Could you check a few things on this model? Use its own coordinates, in mm. A direction names the side the tool comes from. Give positions to 0.01 mm unless a question says otherwise; leave off trailing zeros. Order: outer loops, then holes, each group sorted by start corner. A loop starts at its lowest first (then second) coordinate and runs counter-clockwise, first axis right, second up. Notation, with made-up numbers: (83.5, 85) - (108.5, 85) arc R18 ccw to (108.5, 102) - close; hole circle Ø2 at (20.5, 78.5). An arc over 180 degrees is marked (long way). Put each result on its own line as item: value.
from build123d import *

# Parameters (mm, degrees)
SKETCH1_W           = 53
SKETCH1_H           = 61
BOSS_EXTRUDE1_DEPTH = 5
SKETCH2_W           = 5
SKETCH2_H           = 34
BOSS_EXTRUDE2_DEPTH = 5
SKETCH3_W           = 53
SKETCH3_H           = 5
BOSS_EXTRUDE3_DEPTH = 3
SKETCH4_W           = 53
SKETCH4_H           = 3
BOSS_EXTRUDE4_DEPTH = 8
SKETCH5_W           = 53
SKETCH5_H           = 3
BOSS_EXTRUDE5_DEPTH = 3
CUT_EXTRUDE1_REACH  = 83.847
SKETCH6_W           = 19.5
SKETCH6_H           = 6
CHAMFER1_SIZE       = 0.5
FILLET1_R           = 2.5
SKETCH7_R           = 15
CUT_EXTRUDE2_DEPTH  = 5
FILLET2_R           = 3
SKETCH8_W           = 39
SKETCH8_H           = 3
BOSS_EXTRUDE6_DEPTH = 3
SKETCH10_R          = 1.9
BOSS_EXTRUDE7_DEPTH = 4
FILLET3_START       = 4
FILLET3_DEPTH       = 2
FILLET3_2_DEPTH     = 5
FILLET3_START_2     = 10
FILLET3_3_DEPTH     = 34.381943016
SKETCH11_R          = 1.9
CUT_EXTRUDE3_DEPTH  = 5


with BuildPart() as part:
    # Sketch1 → Boss-Extrude1 (new body)
    with BuildSketch(Plane(origin=(0, 0, 0), x_dir=(1, 0, 0), z_dir=(0, 1, 0))):
        with Locations((26.5, -30.5)):
            Rectangle(SKETCH1_W, SKETCH1_H)
    extrude(amount=BOSS_EXTRUDE1_DEPTH)

    # Sketch2 → Boss-Extrude2 (add)
    with BuildSketch(Plane(origin=(0, 5, 0), x_dir=(1, 0, 0), z_dir=(0, 1, 0))):
        with Locations((2.5, -27)):
            Rectangle(SKETCH2_W, SKETCH2_H)
        with Locations((50.5, -27)):
            Rectangle(SKETCH2_W, SKETCH2_H)
    extrude(amount=BOSS_EXTRUDE2_DEPTH)

    # Sketch3 → Boss-Extrude3 (add)
    with BuildSketch(Plane(origin=(0, 0, 0), x_dir=(-1, 0, 0), z_dir=(0, 0, -1))):
        with Locations((-26.5, 2.5)):
            Rectangle(SKETCH3_W, SKETCH3_H)
    extrude(amount=BOSS_EXTRUDE3_DEPTH)

    # Sketch4 → Boss-Extrude4 (add)
    with BuildSketch(Plane(origin=(0, 5, 0), x_dir=(1, 0, 0), z_dir=(0, 1, 0))):
        with Locations((26.5, 1.5)):
            Rectangle(SKETCH4_W, SKETCH4_H)
    extrude(amount=BOSS_EXTRUDE4_DEPTH)

    # Sketch5 → Boss-Extrude5 (add)
    with BuildSketch(Plane.XY):
        with Locations((26.5, 11.5)):
            Rectangle(SKETCH5_W, SKETCH5_H)
    extrude(amount=BOSS_EXTRUDE5_DEPTH)

    # Cut-Extrude1: up to this face of the body (flat: up to its plane)
    cut_extrude1_end = Plane(part.part.faces().sort_by_distance((26.5, 5, 30.911337712))[0])
    # Sketch6 → Cut-Extrude1 (cut, up to the picked face)
    with BuildSketch(Plane(origin=(0, 13, 0), x_dir=(1, 0, 0), z_dir=(0, 1, 0)), mode=Mode.PRIVATE) as cut_extrude1_sk1:
        with Locations((36.25, 0)):
            Rectangle(SKETCH6_W, SKETCH6_H)
    cut_extrude1_tool1 = split(extrude(cut_extrude1_sk1.sketch, amount=-CUT_EXTRUDE1_REACH, mode=Mode.PRIVATE), bisect_by=cut_extrude1_end, keep=Keep.BOTH, mode=Mode.PRIVATE)
    # Sketch6 → Cut-Extrude1 (cut, up to the picked face)
    with BuildSketch(Plane(origin=(0, 13, 0), x_dir=(1, 0, 0), z_dir=(0, 1, 0)), mode=Mode.PRIVATE) as cut_extrude1_sk2:
        with Locations((16.75, 0)):
            Rectangle(SKETCH6_W, SKETCH6_H)
    cut_extrude1_tool2 = split(extrude(cut_extrude1_sk2.sketch, amount=-CUT_EXTRUDE1_REACH, mode=Mode.PRIVATE), bisect_by=cut_extrude1_end, keep=Keep.BOTH, mode=Mode.PRIVATE)
    add(cut_extrude1_tool1.solids().sort_by(Axis((36.25, 13, 0), (0, -1, 0)))[0], mode=Mode.SUBTRACT)
    add(cut_extrude1_tool2.solids().sort_by(Axis((16.75, 13, 0), (0, -1, 0)))[0], mode=Mode.SUBTRACT)

    # Chamfer1
    chamfer1_edges = [part.edges().sort_by_distance(p)[0] for p in [
        (2.5, 10, 10),
        (2.5, 10, 44),
        (50.5, 10, 44),
        (50.5, 10, 10),
    ]]
    chamfer(chamfer1_edges, length=CHAMFER1_SIZE)

    # Fillet1
    fillet1_edges = [part.edges().sort_by_distance(p)[0] for p in [
        (3.5, 13, -3),
        (49.5, 13, -3),
    ]]
    fillet(fillet1_edges, radius=FILLET1_R)

    # Sketch7 → Cut-Extrude2 (cut)
    with BuildSketch(Plane(origin=(0, 5, 0), x_dir=(1, 0, 0), z_dir=(0, 1, 0))):
        with Locations(Location((26.5, -22, 0), (0, 0, 270))):
            Circle(SKETCH7_R)
    extrude(amount=-CUT_EXTRUDE2_DEPTH, mode=Mode.SUBTRACT)

    # Fillet2
    fillet2_edges = [part.edges().sort_by_distance(p)[0] for p in [
        (53, 2.5, 61),
        (0, 2.5, 61),
    ]]
    fillet(fillet2_edges, radius=FILLET2_R)

    # Sketch8 → Boss-Extrude6 (add)
    with BuildSketch(Plane(origin=(0, 5, 0), x_dir=(1, 0, 0), z_dir=(0, 1, 0))):
        with Locations((26.5, 1.5)):
            Rectangle(SKETCH8_W, SKETCH8_H)
    extrude(amount=BOSS_EXTRUDE6_DEPTH)

    # Sketch10 → Boss-Extrude7 (add)
    # profile 1 of 2: a face of its own
    with BuildSketch(Plane.XZ):
        with BuildLine():
            Line((53, 12.5), (53, 42.5))
            ThreePointArc((53, 42.5), (68, 27.5), (53, 12.5))
        make_face()
        with Locations(Location((61, 27.5, 0), (0, 0, 90))):
            Circle(SKETCH10_R, mode=Mode.SUBTRACT)
    # profile 2 of 2: a face of its own
    with BuildSketch(Plane.XZ):
        with BuildLine():
            Line((0, 12.5), (0, 42.5))
            ThreePointArc((0, 42.5), (-15, 27.5), (0, 12.5))
        make_face()
        with Locations(Location((-8, 27.5, 0), (0, 0, 270))):
            Circle(SKETCH10_R, mode=Mode.SUBTRACT)
    extrude(amount=-BOSS_EXTRUDE7_DEPTH)

    # Fillet3: read off the stored shape, not the designer's step
    # Fillet3 outline → Fillet3 (add)
    with BuildSketch(Plane(origin=(0, 0, 0), x_dir=(1, 0, 0), z_dir=(0, 1, 0)).offset(FILLET3_START)):
        with BuildLine():
            ThreePointArc((0, -10.618056984), (-0.504909997, -11.946479312), (-1.764705882, -12.604167927))
            ThreePointArc((-1.764705882, -12.604167927), (-15, -27.5), (-1.764705882, -42.395832073))
            ThreePointArc((-1.764705882, -42.395832073), (-0.639238058, -42.916225808), (-0.03680884, -44))
            Line((-0.03680884, -44), (0, -44))
            Line((0, -44), (0, -10.618056984))
        make_face()
        with BuildLine():
            Line((53, -44), (53.03680884, -44))
            ThreePointArc((53.03680884, -44), (53.639238058, -42.916225808), (54.764705882, -42.395832073))
            ThreePointArc((54.764705882, -42.395832073), (68, -27.5), (54.764705882, -12.604167927))
            ThreePointArc((54.764705882, -12.604167927), (53.504909997, -11.946479312), (53, -10.618056984))
            Line((53, -10.618056984), (53, -44))
        make_face()
    extrude(amount=FILLET3_DEPTH)

    # Fillet3 2 outline → Fillet3 2 (add)
    with BuildSketch(Plane(origin=(0, 0, 0), x_dir=(1, 0, 0), z_dir=(0, 1, 0))):
        with BuildLine():
            Line((0, -12.5), (0, -10.618056984))
            ThreePointArc((0, -10.618056984), (-0.504909997, -11.946479312), (-1.764705882, -12.604167927))
            ThreePointArc((-1.764705882, -12.604167927), (-0.883888823, -12.526064627), (0, -12.5))
        make_face()
        with BuildLine():
            ThreePointArc((0, -42.5), (-0.883888823, -42.473935373), (-1.764705882, -42.395832073))
            ThreePointArc((-1.764705882, -42.395832073), (-0.504909997, -43.053520688), (0, -44.381943016))
            Line((0, -44.381943016), (0, -42.5))
        make_face()
        with BuildLine():
            ThreePointArc((53, -44.381943016), (53.504909997, -43.053520688), (54.764705882, -42.395832073))
            ThreePointArc((54.764705882, -42.395832073), (53.883888823, -42.473935373), (53, -42.5))
            Line((53, -42.5), (53, -44.381943016))
        make_face()
        with BuildLine():
            ThreePointArc((53, -12.5), (53.883888823, -12.526064627), (54.764705882, -12.604167927))
            ThreePointArc((54.764705882, -12.604167927), (53.504909997, -11.946479312), (53, -10.618056984))
            Line((53, -10.618056984), (53, -12.5))
        make_face()
    extrude(amount=FILLET3_2_DEPTH)

    # Fillet3 3 outline → Fillet3 3 (cut)
    with BuildSketch(Plane.XY.offset(FILLET3_START_2)):
        with BuildLine():
            Line((-16, 4), (-2, 4))
            ThreePointArc((-2, 4), (-0.585786438, 4.585786438), (0, 6))
            Line((0, 6), (-16, 6))
            Line((-16, 6), (-16, 4))
        make_face()
        with BuildLine():
            ThreePointArc((53, 6), (53.585786438, 4.585786438), (55, 4))
            Line((55, 4), (69, 4))
            Line((69, 4), (69, 6))
            Line((69, 6), (53, 6))
        make_face()
    extrude(amount=FILLET3_3_DEPTH, mode=Mode.SUBTRACT)

    # Sketch11 → Cut-Extrude3 (cut)
    with BuildSketch(Plane(origin=(0, 5, 0), x_dir=(1, 0, 0), z_dir=(0, 1, 0))):
        with Locations(Location((5, -57.5, 0), (0, 0, 270))):
            Circle(SKETCH11_R)
        with Locations(Location((48, -57.5, 0), (0, 0, 270))):
            Circle(SKETCH11_R)
    extrude(amount=-CUT_EXTRUDE3_DEPTH, mode=Mode.SUBTRACT)


solid = part.part
1) Suppose I cut it at D-D, the plane x = 44. List the corners of the cut face in (y, z) for me, and give its area (3 significant figures).
Filled in:
outline: (0, -3) - (8, -3) - (8, 0) - (5, 0) - (5, 61) - (0, 61) - close
area: 329 mm^2
2) Which directions (+Z, -Z, +X, -X, +Y, -Y) give clear straight access to the entire face, cutting with the end or side of a thin tool? Please do faces 4 (the flat face through (46, 11, 0)), 5 (the flat face through (26, 7, 0)), 6 (the flat face through (53, 2, 51)), 7 (the flat face through (49, 12, 3)).
Filled in:
face 4: +Z, -Z, +Y
face 5: +X, -X
face 6: +Z, +X, +Y, -Y
face 7: +Z, +X, -X, +Y
3) Suppose I cut it at A-A, the plane x = 26.5. List the corners of the cut face in (y, z) for me.
Filled in:
outline: (0, -3) - (8, -3) - (8, 0) - (5, 0) - (5, 7) - (0, 7) - close; (0, 37) - (5, 37) - (5, 61) - (0, 61) - close
4) Suppose I cut it at C-C, the plane z = 28. List the corners of the cut face in (x, y) for me, and give its area (3 significant figures).
Filled in:
outline: (-14.99, 0) - (-9.83, 0) - (-9.83, 4) - (-14.99, 4) - close; (-6.17, 0) - (12.75, 0) - (12.75, 5) - (5, 5) - (5, 10) - (0, 10) - (0, 6) arc R2 cw to (-2, 4) - (-6.17, 4) - close; (40.25, 0) - (59.17, 0) - (59.17, 4) - (55, 4) arc R2 cw to (53, 6) - (53, 10) - (48, 10) - (48, 5) - (40.25, 5) - close; (62.83, 0) - (67.99, 0) - (67.99, 4) - (62.83, 4) - close
area: 270 mm^2
5) If I drill on line 1 (X direction, y = 1.35, z = 57.5); line 2 (X direction, y = 1.8, z = 27.5); line 3 (Y direction, x = 41.5, z = 33.5), over which ranges is the centre line in solid material (lowest first)? Write a range as [from, to].
Filled in:
line 1: x = [0, 3.1], [6.9, 46.1], [49.9, 53]
line 2: x = [-15, -9.9], [-6.1, 12.54], [40.46, 59.1], [62.9, 68]
line 3: y = [0, 5]
6) I'm going to push flat-ended pins straight in: pin 1 (4 mm diameter, centred on x = 51.5, z = 53, fed in from +Y); pin 2 (4 mm diameter, centred on x = 63.5, z = 21.5, fed in from +Y); pin 3 (1.5 mm diameter, centred on y = 11, z = -1, fed in from +X). Where does each tip first touch, or does it pass through?
Filled in:
pin 1: stops at y = 5
pin 2: stops at y = 4
pin 3: stops at x = 53
7) We'd pull the mould along Z, two halves only. Please class faces 1 (the flat face through (35, 0, 36)), 2 (the cylindrical face through (62.686, 1.972, 28.377)), 3 (the cylindrical face through (-0.518, 2.145, 43.038)): pulls with the +Z half, pulls with the -Z half, needs draft (parallel to the pull), parting line crosses it, or undercut.
Filled in:
face 1: needs draft
face 2: undercut
face 3: pulls with the +Z half
8) Suppose I cut it at B-B, the plane y = 2.5. List the corners of the cut face in (x, z) for me, and give its area (3 significant figures).
Filled in:
outline: (-1.76, 12.6) arc R2 cw to (0, 10.62) - (0, -3) - (53, -3) - (53, 10.62) arc R2 cw to (54.76, 12.6) arc R15 ccw to (54.76, 42.4) arc R2 cw to (53, 44.38) - (53, 58) arc R3 ccw to (50, 61) - (3, 61) arc R3 ccw to (0, 58) - (0, 44.38) arc R2 cw to (-1.76, 42.4) arc R15 ccw to start; hole circle Ø3.8 at (-8, 27.5); hole circle Ø3.8 at (5, 57.5); hole circle Ø30 at (26.5, 22); hole circle Ø3.8 at (48, 57.5); hole circle Ø3.8 at (61, 27.5)
area: 3,350 mm^2
